Build history of the part. All positions in model axes, mm. Face numbers are marked on the shaded views. A direction names the side the tool comes from. Round coordinates to 2 decimals unless told otherwise and drop trailing zeros. Write each loop counter-clockwise with the first axis right and the second up, starting at its lowest first coordinate (ties: lowest second). Pieces come first, ordered by that corner, then holes. Notation, with made-up numbers: (-6, 83) - (3, 83) arc R19 ccw to (3, 92) - close; hole circle Ø1 at (33, -12). An arc over 180 degrees is marked (long way). Answer as a JSON object with one key per item and string values. Group by question number.
Item 1: Which spindle directions (+Z, -Z, +X, -X, +Y, -Y) get a long thin tool onto all of the face, cutting with end or side? Do the marked faces 1, 2, 3, 4 and 5. Say none if no direction does.
Item 2: Slice it at A-A, the plane y = 34. List the corners of the cut face in (x, z), then the cut area to 4 significant figures.
Item 3: Slice it at D-D, the plane y = 0. List the corners of the cut face in (x, z).
Item 4: Two-plate mould, pull along X, no slides. Class the marked faces 6, 7 and 8: +X half, -X half, draft (parallel to the pull), parting line (faces both ways), or undercut.
Item 5: Flat gauge pins, fed straight in: pin 1 (2 mm diameter, centred on y = 16, z = 5, fed in from -X); pin 2 (1 mm diameter, centred on y = 34, z = 1.5, fed in from -X); pin 3 (0.6 mm diameter, centred on x = -15, z = 6, fed in from +Y). Where does each tip first touch, or does it go through?
Item 6: Slice it at B-B, the plane x = -12. List the corners of the cut face in (y, z).
Item 7: Probe line 1 (Y direction, x = 0, z = 1.2); line 2 (Y direction, x = -5, z = 1.5); line 3 (Y direction, x = -11, z = 10). List the from-to ranges inside material, lowest first. Write a range as from..to.
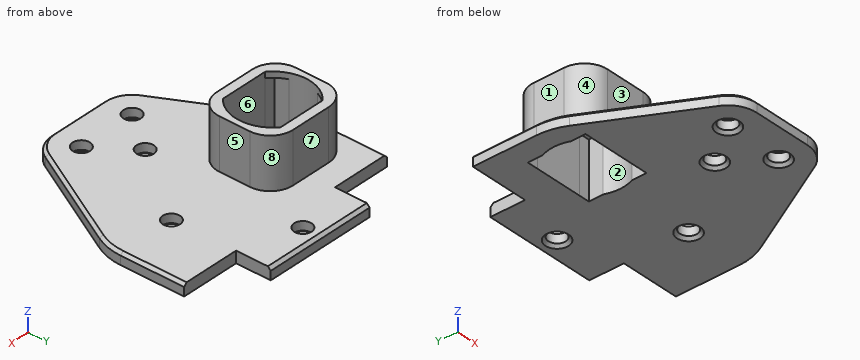
Solid Edge part; units mm, degrees
sketch "Sketch1" plane through (0, 0, 0) normal (0, 0, 1) x (1, 0, 0)
  line L0 (-9.4118, -2.3529) -> (-18.8235, 15.2941)
  arc A0 (-18.8235, 15.2941) -> (-20, 20) centre (-10, 20) cw
  line L1 (-20, 20) -> (-20, 31)
  line L2 (-20, 31) -> (-9.75, 31)
  line L3 (-9.75, 37) -> (-9.75, 31)
  line L4 (-9.75, 37) -> (9.75, 37)
  line L5 (9.75, 37) -> (9.75, 31)
  line L6 (9.75, 31) -> (20, 31)
  line L7 (20, 31) -> (20, 20)
  arc A1 (20, 20) -> (18.8235, 15.2941) centre (10, 20) cw
  line L8 (9.4118, -2.3529) -> (18.8235, 15.2941)
  line L9 (-5, -5) -> (5, -5)
  arc A2 (9.4118, -2.3529) -> (5, -5) centre (5, 0) cw
  arc A3 (-5, -5) -> (-9.4118, -2.3529) centre (-5, 0) cw
  circle A4 centre (10, 20) radius 1.5
  circle A5 centre (5, 0) radius 1.5
  circle A6 centre (-5, 0) radius 1.5
  circle A7 centre (0, 6.6667) radius 1.5
extrude "Protrusion1" add sketch "Sketch1" along normal blind 2
sketch "Sketch2" plane through (0, 0, 0) normal (0, 0, 1) x (1, 0, 0)
  line L0 (-17.5, 26.6144) -> (-17.5, 13.3856)
  line L1 (-17.5, 13.3856) -> (-2.5, 13.3856)
  line L2 (-2.5, 13.3856) -> (-2.5, 26.6144)
  line L3 (-2.5, 26.6144) -> (-17.5, 26.6144)
extrude "Protrusion2" add sketch "Sketch2" along normal blind 10.75
sketch "Sketch3" plane through (0, 0, 0) normal (0, 0, 1) x (1, 0, 0)
  line L0 (-16, 25) -> (-16, 15)
  line L1 (-16, 15) -> (-4, 15)
  line L2 (-4, 15) -> (-4, 25)
  line L3 (-4, 25) -> (-16, 25)
extrude "VaciadoExtruido_2" cut sketch "Sketch3" along normal blind 9.75
sketch "Sketch4" plane through (-10, 20, 10.75) normal (0, 0, 1) x (1, 0, 0)
  line L0 (-4.1533, 5) -> (4.1533, 5)
  arc A0 (4.1533, 5) -> (4.1533, -5) centre (0, 0) cw
  line L1 (-4.1533, -5) -> (4.1533, -5)
  arc A1 (-4.1533, -5) -> (-4.1533, 5) centre (0, 0) cw
extrude "Cutout1" cut sketch "Sketch4" against normal through all
fillet "Redondeo_1" radius 4 4 edges at (-2.5, 13.3856, 6.375) (-17.5, 13.3856, 6.375) (-17.5, 26.6144, 6.375) (-2.5, 26.6144, 6.375)
chamfer "Chaflán_1" distance 0.5 angle 45 10 edges at (0, -5, 2) (-7.5725, -4.2875, 2) (-14.1176, 6.4706, 2) (14.1176, 6.4706, 2) (7.5725, -4.2875, 2) (19.7014, 17.5746, 2) (20, 25.5, 2) (-19.7014, 17.5746, 2) (-20, 25.5, 2) (0, 37, 2)
sketch "Sketch5" plane through (0, 0, 0) normal (0, 0, 1) x (1, 0, 0)
  circle A0 centre (0, 34) radius 1.5
extrude "Cutout2" cut sketch "Sketch5" along normal through all
chamfer "Chaflán_2" distance 0.5 angle 45 4 edges at (8.5, 20, 0) (3.5, 0, 0) (-6.5, 0, 0) (-1.5, 34, 0)
chamfer "Chaflán_3" distance 0.5 angle 45 1 edges at (-1.5, 6.6667, 0)
Geometry says:
{
 "1": {"face 1": "+Z, -X, +Y, -Y", "face 2": "+Z, -Z", "face 3": "+Z, +X, -X, -Y", "face 4": "+Z, -X, -Y", "face 5": "+Z, +X, +Y, -Y"},
 "2": {"outline": "(-9.75, 0) - (-2, 0) - (-1.5, 0.5) - (-1.5, 2) - (-9.75, 2) - close; (1.5, 0.5) - (2, 0) - (9.75, 0) - (9.75, 2) - (1.5, 2) - close", "area": "32.75 mm^2"},
 "3": {"outline": "(-10.67, 0) - (-7, 0) - (-6.5, 0.5) - (-6.5, 2) - (-10.1, 2) - (-10.67, 1.5) - close; (-3.5, 0.5) - (-3, 0) - (3, 0) - (3.5, 0.5) - (3.5, 2) - (-3.5, 2) - close; (6.5, 0.5) - (7, 0) - (10.67, 0) - (10.67, 1.5) - (10.1, 2) - (6.5, 2) - close"},
 "4": {"face 6": "undercut", "face 7": "draft", "face 8": "+X half"},
 "5": {"pin 1": "stops at x = -17.48", "pin 2": "stops at x = -9.75", "pin 3": "stops at y = 26.43"},
 "6": {"outline": "(2.5, 0) - (15, 0) - (15, 10.75) - (13.39, 10.75) - (13.39, 2) - (3.56, 2) - (2.5, 1.5) - close; (25, 0) - (31, 0) - (31, 2) - (26.61, 2) - (26.61, 10.75) - (25, 10.75) - close"},
 "7": {"line 1": "y = -5..5.17, 8.17..32.5, 35.5..37", "line 2": "y = -5..-1.5, 1.5..15, 25..37", "line 3": "y = 13.39..15, 25..26.61"}
}
